from build123d import *

# Parameters (mm, degrees)
F0_R     = 9
F0_R_2   = 2
F1_DEPTH = 12
F2_R     = 76.2
F3_DEPTH = 38.8
F5_R     = 2
F6_DEPTH = 12


with BuildPart() as f1:
    # F0 (on Top) → F1 (new body)
    with BuildSketch(Plane.XY):
        with Locations((0.035375, -0.025554)):
            Circle(F0_R)
        with Locations((0.035375, -0.025554)):
            Circle(F0_R_2, mode=Mode.SUBTRACT)
    extrude(amount=-F1_DEPTH)

    # F2 (on Top) → F3 (join)
    with BuildSketch(Plane.XY):
        Circle(F2_R)
    extrude(amount=-F3_DEPTH)

    # F5 (on face) → F6 (cut)
    with BuildSketch(Plane.XY):
        Circle(F5_R)
    extrude(amount=-F6_DEPTH, mode=Mode.SUBTRACT)


solid = f1.part
The listing builds one solid part. Answer for the finished solid, in the listing's coordinates (mm). A direction names the side the tool comes from. Give positions to 0.01 mm unless a question says otherwise; leave off trailing zeros. Write each loop counter-clockwise with the first axis right and the second up, starting at its lowest first coordinate (ties: lowest second). Pieces come first, ordered by that corner, then holes.
Item 1: Find the intervals of material crossed by line 1 along Y through (x, z) = (0, -4.75); line 2 along Y through (x, z) = (42, -26.5); line 3 along Y through (x, z) = (-14, -23.5), in increasing order.
Item 2: Which of the six approach directions +Z, -Z, +X, -X, +Y, -Y give full straight-line access (tool end or side, diameter ignored) to faces 4 (the flat face through (16, 1, 0)), 5 (the flat face through (0, 0, -12))?
Item 3: Flat-ended cylindrical pins translate along their axes: P1, Ø12, axis at y = -50.5, z = -17, coming from the +X side; P2, Ø4.5, axis at x = 0, y = 0.5, coming from the +Z side; P3, Ø2, axis at y = 41, z = -14.5, coming from the +X side; P4, Ø2, axis at x = -9.5, z = -30, coming from the +Y side. Find the tip coordinate at first contact, or state that the pin passes through.
Item 4: Determine the mould class of faces 1 (the cylindrical face through (-60.47, -46.367, -19.128)), 2 (the cylindrical face through (0, -2, -6)), 3 (the flat face through (-1, 1, -38.8)) for opening direction X: released by +X, released by -X, zero draft, split by the parting line, or undercut.
Item 5: Section A-A, the plane z = -21 is taken. Write down the section's boundary in (x, y), plus the area to 3 significant figures.
Item 6: Section B-B, the plane x = 40.5 is taken. Write down the section's boundary in (y, z).
Item 7: Section C-C, the plane y = 27 is taken. Write down the section's boundary in (x, z).
Completed:
1. line 1: y = -76.2 to -2, 2 to 76.2
1. line 2: y = -63.58 to 63.58
1. line 3: y = -74.9 to 74.9
2. face 4: +Z, +X, -X, +Y, -Y
2. face 5: +Z
3. P1: stops at x = 61.86
3. P2: stops at z = 0
3. P3: stops at x = 64.86
3. P4: stops at y = 75.72
4. face 1: split by the parting line
4. face 2: undercut
4. face 3: zero draft
5. outline: circle Ø152.4 at (0, 0)
5. area: 18,200 mm2
6. outline: (-64.55, -38.8) - (64.55, -38.8) - (64.55, 0) - (-64.55, 0) - close
7. outline: (-71.26, -38.8) - (71.26, -38.8) - (71.26, 0) - (-71.26, 0) - close
